```python
from build123d import *

# Parameters (mm, degrees)
F0_R     = 1.8
F1_DEPTH = 3
F2_R     = 1.25
F3_DEPTH = 3.001


with BuildPart() as f1:
    # F0 (on Top) → F1 (new body)
    with BuildSketch(Plane.XY):
        with BuildLine():
            Line((63, 75), (-63, 75))
            ThreePointArc((-63, 75), (-71.485281, 71.485281), (-75, 63))
            Line((-75, 63), (-75, -63))
            ThreePointArc((-75, -63), (-71.485281, -71.485281), (-63, -75))
            Line((-63, -75), (63, -75))
            ThreePointArc((63, -75), (71.485281, -71.485281), (75, -63))
            Line((75, -63), (75, 63))
            ThreePointArc((75, 63), (71.485281, 71.485281), (63, 75))
        make_face()
        with Locations((-47.266874, -62.823223)):
            Circle(F0_R, mode=Mode.SUBTRACT)
        with Locations((-62.823223, -47.266874)):
            Circle(F0_R, mode=Mode.SUBTRACT)
        Polygon((-58.757359, -67.242641), (-67.242641, -58.757359), (-51.332738, -42.847457), (-42.847457, -51.332738), align=None, mode=Mode.SUBTRACT)
        with Locations((47.266874, -62.823223)):
            Circle(F0_R, mode=Mode.SUBTRACT)
        Polygon((42.847457, -51.332738), (51.332738, -42.847457), (67.242641, -58.757359), (58.757359, -67.242641), align=None, mode=Mode.SUBTRACT)
        with Locations((62.823223, -47.266874)):
            Circle(F0_R, mode=Mode.SUBTRACT)
        with Locations((-62.823223, 47.266874)):
            Circle(F0_R, mode=Mode.SUBTRACT)
        Polygon((-67.242641, 58.757359), (-58.757359, 67.242641), (-42.847457, 51.332738), (-51.332738, 42.847457), align=None, mode=Mode.SUBTRACT)
        with Locations((-47.266874, 62.823223)):
            Circle(F0_R, mode=Mode.SUBTRACT)
        with BuildLine():
            Line((-40, -35), (-40, 0))
            Line((-40, 0), (-40, 35))
            ThreePointArc((-40, 35), (-38.535534, 38.535534), (-35, 40))
            Line((-35, 40), (0, 40))
            Line((0, 40), (35, 40))
            ThreePointArc((35, 40), (38.535534, 38.535534), (40, 35))
            Line((40, 35), (40, 0))
            Line((40, 0), (40, -35))
            ThreePointArc((40, -35), (38.535534, -38.535534), (35, -40))
            Line((35, -40), (0, -40))
            Line((0, -40), (-35, -40))
            ThreePointArc((-35, -40), (-38.535534, -38.535534), (-40, -35))
        make_face(mode=Mode.SUBTRACT)
        Polygon((51.332738, 42.847457), (42.847457, 51.332738), (58.757359, 67.242641), (67.242641, 58.757359), align=None, mode=Mode.SUBTRACT)
        with Locations((62.823223, 47.266874)):
            Circle(F0_R, mode=Mode.SUBTRACT)
        with Locations((47.266874, 62.823223)):
            Circle(F0_R, mode=Mode.SUBTRACT)
    extrude(amount=F1_DEPTH)

    # F2 (on face) → F3 (cut, through all)
    with BuildSketch(Plane.XY.offset(3)):
        with Locations((-64.80856, -64.80856)):
            Circle(F2_R)
        with Locations((-45.123414, -45.123414)):
            Circle(F2_R)
        with Locations((45.123414, -45.123414)):
            Circle(F2_R)
        with Locations((45.123414, 45.123414)):
            Circle(F2_R)
        with Locations((-45.123414, 45.123414)):
            Circle(F2_R)
        with Locations((64.80856, -64.80856)):
            Circle(F2_R)
        with Locations((64.80856, 64.80856)):
            Circle(F2_R)
        with Locations((-64.80856, 64.80856)):
            Circle(F2_R)
    extrude(amount=-F3_DEPTH, mode=Mode.SUBTRACT)


with BuildPart() as f4_1:
    # F4: copy of F1
    add(f1.part.moved(Location((0, 0, 20))))


solid = f1.part
```
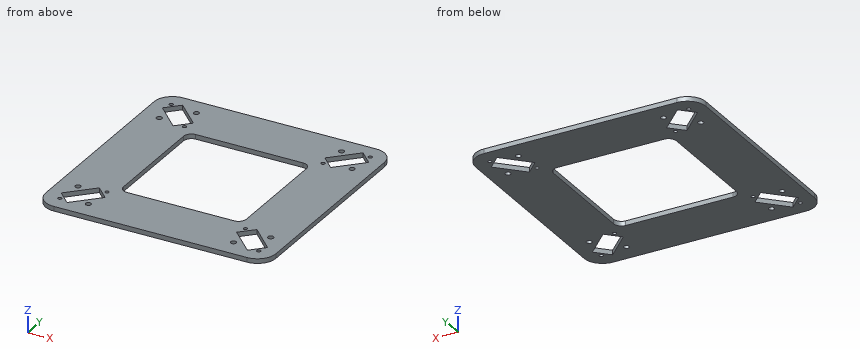
For this review, take the finished solid that the model builds, in its own axes (mm). Coordinates: 2 decimals unless noted, no trailing zeros. Write each loop counter-clockwise with the first axis right and the second up, starting at its lowest first coordinate (ties: lowest second). Pieces come first, ordered by that corner, then holes. Notation, with made-up numbers: (-6, -39) - (7, -39) arc R19 cw to (7, -35) - close; hole circle Ø7 at (-28.5, 85). An arc over 180 degrees is marked (long way). Answer in a Markdown table with one row per item. Add a question column.
Q1. For P1, Ø4, axis at x = -41, y = -53, coming from the -Z side; P2, Ø3, axis at x = 47.27, y = -62.82, coming from the -Z side, all flat-tipped, find the tip position at first contact; note any pin that passes through.
Q2. We need section A-A, the plane x = 31.5. State the section outline as (y, z) points, and give its area (3 significant figures).
Q3. For probe 1 along Y at (x, z) = (22, 0.2); probe 2 along X at (y, z) = (-57, 0.85), list the stretches that pass through material, from the lowest coordinate up.
Q4. We need section C-C, the plane z = 1.1. Count the separate pieces of the cut face and the enclosed holes in it, and give its area (3 significant figures).
Answer list:
| question | item | result |
|---|---|---|
| 1 | P1 | stops at z = 0 |
| 1 | P2 | passes through |
| 2 | outline | (-75, 0) - (-40, 0) - (-40, 3) - (-75, 3) - close; (40, 0) - (75, 0) - (75, 3) - (40, 3) - close |
| 2 | area | 210 mm2 |
| 3 | probe 1 | y = -75 to -40, 40 to 75 |
| 3 | probe 2 | x = -75 to -65.49, -48.51 to 48.51, 65.49 to 75 |
| 4 | separate pieces | 1 |
| 4 | enclosed holes | 21 |
| 4 | area | 14,800 mm2 |
